The listing builds one solid part. Answer for the finished solid, in the listing's coordinates (mm). Face numbers are marked on the shaded views. A direction names the side the tool comes from. Coordinates: 2 decimals unless noted, no trailing zeros. Write each loop counter-clockwise with the first axis right and the second up, starting at its lowest first coordinate (ties: lowest second). Pieces come first, ordered by that corner, then holes.
(1) Which of the six approach directions +Z, -Z, +X, -X, +Y, -Y give full straight-line access (tool end or side, diameter ignored) to the marked faces 1 and 2?
(2) The part is cut by section C-C on x = 115. Determine the outline of the cut face in (y, z).
(3) The part is cut by section B-B on x = 239. Determine the outline of the cut face in (y, z).
(4) Given P1, Ø5, axis at x = 304, y = 0, coming from the -Z side; P2, Ø10, axis at x = 133.5, z = 7.5, coming from the -Y side; P3, Ø1, axis at x = -12.5, y = 3.5, coming from the +Z side, each flat-ended and moving along its own axis, determine where each tip first touches the part or whether it passes through.
(5) Straight lines are drawn through the part: line 1 (X direction, y = 12.5, z = 7.5); line 2 (Z direction, x = 34, y = 15); line 3 (Y direction, x = -188, z = 1). For each, find the intervals that lie inside material, in ascending order.
(6) The part is cut by section A-A on z = 5.5. Determine the outline of the cut face in (x, y), plus the area to 3 significant figures.
from build123d import *

# Parameters (mm, degrees)
CUT_EXTRUDE1_DEPTH = 431
CUT_EXTRUDE2_DEPTH = 4
SKETCH4_W          = 1.6
SKETCH4_H          = 0.7
CUT_EXTRUDE3_DEPTH = 5


with BuildPart() as part:
    # Sketch1 → Revolve1 (revolve)
    with BuildSketch(Plane.XY, mode=Mode.PRIVATE) as revolve1_sk:
        Polygon((-337.5, 0), (337.5, 0), (337.5, 15), (213.5, 15), (213.5, 17.5), (-217.5, 17.5), (-217.5, 15), (-337.5, 15), align=None)
    revolve(revolve1_sk.sketch.rotate(Axis((-337.5, 0, 0), (1, 0, 0)), 90), axis=Axis((-337.5, 0, 0), (1, 0, 0)))

    # Sketch2 → Cut-Extrude1 (cut)
    with BuildSketch(Plane.ZY.offset(217.5)):
        with BuildLine():
            Line((-14.936600675, 9.118550338), (-15.062665819, -8.908765258))
            ThreePointArc((-15.062665819, -8.908765258), (-17.499572122, 0.12237463), (-14.936600675, 9.118550338))
        make_face()
        with BuildLine():
            Line((14.936600675, 9.118550338), (15.062665819, -8.908765258))
            ThreePointArc((15.062665819, -8.908765258), (17.499572122, 0.12237463), (14.936600675, 9.118550338))
        make_face()
    extrude(amount=-CUT_EXTRUDE1_DEPTH, mode=Mode.SUBTRACT)

    # Sketch3 → Cut-Extrude2 (cut)
    with BuildSketch(Plane.XY.offset(-15)):
        with BuildLine():
            Line((-331.5, 4), (-311.5, 4))
            ThreePointArc((-311.5, 4), (-307.5, 0), (-311.5, -4))
            Line((-311.5, -4), (-331.5, -4))
            ThreePointArc((-331.5, -4), (-335.5, 0), (-331.5, 4))
        make_face()
    extrude(amount=CUT_EXTRUDE2_DEPTH, mode=Mode.SUBTRACT)

    # Sketch4 → Cut-Revolve1 (revolve, cut)
    with BuildSketch(Plane.XY, mode=Mode.PRIVATE) as cut_revolve1_sk:
        with Locations((333.7, 14.65)):
            Rectangle(SKETCH4_W, SKETCH4_H)
    revolve(cut_revolve1_sk.sketch.rotate(Axis((337.5, 0, 0), (-1, 0, 0)), 270.400663256), axis=Axis((337.5, 0, 0), (-1, 0, 0)), mode=Mode.SUBTRACT)

    # Sketch5 → Cut-Extrude3 (cut)
    with BuildSketch(Plane.XY.offset(-15)):
        with BuildLine():
            Line((324.5, -5), (289.5, -5))
            ThreePointArc((289.5, -5), (284.5, 0), (289.5, 5))
            Line((289.5, 5), (324.5, 5))
            ThreePointArc((324.5, 5), (329.5, 0), (324.5, -5))
        make_face()
    extrude(amount=CUT_EXTRUDE3_DEPTH, mode=Mode.SUBTRACT)


solid = part.part
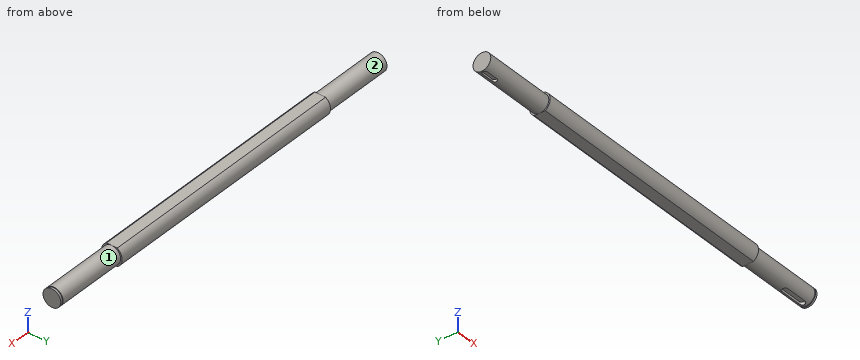
Model answer:
1. face 1: +X
1. face 2: -X
2. outline: (-8.91, -15.06) - (9.12, -14.94) arc R17.5 ccw to (9.12, 14.94) - (-8.91, 15.06) arc R17.5 ccw to start
3. outline: circle Ø30 at (0, 0)
4. P1: stops at z = -10
4. P2: stops at y = -17.32
4. P3: stops at z = 14.98
5. line 1: x = -337.5 to 332.9, 334.5 to 337.5
5. line 2: z = -9.01 to 9.01
5. line 3: y = -17.47 to 17.47
6. outline: (-337.5, -13.96) - (-217.5, -13.96) - (-217.5, -16.61) - (213.5, -16.61) - (213.5, -13.96) - (332.9, -13.96) - (332.9, -13.2) - (334.5, -13.2) - (334.5, -13.96) - (337.5, -13.96) - (337.5, 13.96) - (334.5, 13.96) - (334.5, 13.2) - (332.9, 13.2) - (332.9, 13.96) - (213.5, 13.96) - (213.5, 16.61) - (-217.5, 16.61) - (-217.5, 13.96) - (-337.5, 13.96) - close
6. area: 21,100 mm2
